```python
from build123d import *

# Parameters (mm, degrees)
BOSS_EXTRUDE1_DEPTH = 0.5


with BuildPart() as part:
    # Sketch2 → Boss-Extrude1 (new body)
    with BuildSketch(Plane.XY):
        Polygon((-6.25, -1.4), (-6.25, 1.4), (0.75, 1.4), (0.75, 2.5), (2.25, 2.5), (2.25, 0.6), (3.25, 0.6), (3.25, 0.75), (6.25, 0.2), (6.25, -0.2), (3.25, -0.75), (3.25, -0.6), (2.25, -0.6), (2.25, -2.5), (0.75, -2.5), (0.75, -1.4), align=None)
        with BuildLine():
            Line((-2.875, 0.675), (-4.725, 0.675))
            ThreePointArc((-4.725, 0.675), (-5.4, 0), (-4.725, -0.675))
            Line((-4.725, -0.675), (-2.875, -0.675))
            ThreePointArc((-2.875, -0.675), (-2.2, 0), (-2.875, 0.675))
        make_face(mode=Mode.SUBTRACT)
    extrude(amount=BOSS_EXTRUDE1_DEPTH)


solid = part.part
```
Could you check a few things on this model? Use its own coordinates, in mm. Coordinates: 2 decimals unless noted, no trailing zeros. Write each loop counter-clockwise with the first axis right and the second up, starting at its lowest first coordinate (ties: lowest second). Pieces come first, ordered by that corner, then holes. Notation, with made-up numbers: (87.5, 47.25) - (99.5, 47.25) arc R27 cw to (99.5, 86.25) - close; hole circle Ø11 at (30, -2). An arc over 180 degrees is marked (long way). Use a Markdown table: item, result.
Q1. Imagine slicing it at A-A (z = 0.2). List the corners of the cut face in (x, y) for me (3 decimals), and give its area (3 significant figures).
Geometry check:
| item | result |
|---|---|
| outline | (-6.25, -1.4) - (0.75, -1.4) - (0.75, -2.5) - (2.25, -2.5) - (2.25, -0.6) - (3.25, -0.6) - (3.25, -0.75) - (6.25, -0.2) - (6.25, 0.2) - (3.25, 0.75) - (3.25, 0.6) - (2.25, 0.6) - (2.25, 2.5) - (0.75, 2.5) - (0.75, 1.4) - (-6.25, 1.4) - close; hole (-4.725, -0.675) - (-2.875, -0.675) arc R0.675 ccw to (-2.875, 0.675) - (-4.725, 0.675) arc R0.675 ccw to start |
| area | 27.2 mm2 |
Q2. Imagine slicing it at B-B (y = 0). List the corners of the cut face in (x, z) for me, and give its area (3 significant figures).
Geometry check:
| item | result |
|---|---|
| outline | (-6.25, 0) - (-5.4, 0) - (-5.4, 0.5) - (-6.25, 0.5) - close; (-2.2, 0) - (6.25, 0) - (6.25, 0.5) - (-2.2, 0.5) - close |
| area | 4.65 mm2 |
Q3. Imagine slicing it at D-D (x = 3). List the corners of the cut face in (y, z) for me.
Geometry check:
| item | result |
|---|---|
| outline | (-0.6, 0) - (0.6, 0) - (0.6, 0.5) - (-0.6, 0.5) - close |
Q4. Please list where these lines run through material, in increasing order: L1, parallel to Y at x = 3, z = 0.1; L2, parallel to Y at x = -4.5, z = 0.4 (3 decimals); L3, parallel to X at y = 2.2, z = 0.45.
Geometry check:
| item | result |
|---|---|
| L1 | y = -0.6 to 0.6 |
| L2 | y = -1.4 to -0.675, 0.675 to 1.4 |
| L3 | x = 0.75 to 2.25 |
Q5. Imagine slicing it at C-C (x = -2.5). List the corners of the cut face in (y, z) for me, and give its area (3 significant figures).
Geometry check:
| item | result |
|---|---|
| outline | (-1.4, 0) - (-0.56, 0) - (-0.56, 0.5) - (-1.4, 0.5) - close; (0.56, 0) - (1.4, 0) - (1.4, 0.5) - (0.56, 0.5) - close |
| area | 0.839 mm2 |
